Geometry: final body of the model. Coordinates: model frame, mm. A direction names the side the tool comes from. Give positions to 0.01 mm unless a question says otherwise; leave off trailing zeros. Write each loop counter-clockwise with the first axis right and the second up, starting at its lowest first coordinate (ties: lowest second). Pieces come first, ordered by that corner, then holes.
```python
from build123d import *

# Parameters (mm, degrees)
SKETCH_1_W          = 50
SKETCH_1_H          = 55
EXTRUDE_1_DEPTH     = 8
EXTRUDE_2_DEPTH     = 8
FILLET_1_R          = 8
CUT_EXTRUDE_1_DEPTH = 8
SKETCH_4_R          = 4
CUT_EXTRUDE_2_DEPTH = 8


with BuildPart() as part:
    # 草图1 → 凸台-拉伸1 (new body)
    with BuildSketch(Plane(origin=(0, 0, 0), x_dir=(0, 0, -1), z_dir=(1, 0, 0))):
        with Locations((0, 7.5)):
            Rectangle(SKETCH_1_W, SKETCH_1_H)
    extrude(amount=EXTRUDE_1_DEPTH)

    # 草图2 → 凸台-拉伸2 (add)
    with BuildSketch(Plane.XZ.offset(20)):
        Polygon((0, 25), (8, 25), (246.45, 25), (246.45, -25), (8, -25), (0, -25), align=None)
    extrude(amount=-EXTRUDE_2_DEPTH)

    # 圆角1
    fillet_1_edges = [part.edges().sort_by_distance(p)[0] for p in [
        (8, -12, 0),
    ]]
    fillet(fillet_1_edges, radius=FILLET_1_R)

    # 草图3 → 切除-拉伸1 (cut)
    with BuildSketch(Plane.XZ.offset(20)):
        with BuildLine():
            Line((176.45, -17.75), (226.45, -17.75))
            ThreePointArc((226.45, -17.75), (229.2, -15), (226.45, -12.25))
            Line((226.45, -12.25), (176.450000009, -12.25))
            ThreePointArc((176.450000009, -12.25), (173.7, -14.999999996), (176.45, -17.75))
        make_face()
        with BuildLine():
            Line((176.449999995, 12.25), (226.45, 12.25))
            ThreePointArc((226.45, 12.25), (229.2, 15), (226.45, 17.75))
            Line((226.45, 17.75), (176.45, 17.75))
            ThreePointArc((176.45, 17.75), (173.7, 15.000000003), (176.449999995, 12.25))
        make_face()
    extrude(amount=-CUT_EXTRUDE_1_DEPTH, mode=Mode.SUBTRACT)

    # 草图4 → 切除-拉伸2 (cut)
    with BuildSketch(Plane.ZY):
        with Locations((-15, 25)):
            Circle(SKETCH_4_R)
        with Locations((-15, 0)):
            Circle(SKETCH_4_R)
        with Locations((15, 25)):
            Circle(SKETCH_4_R)
        with Locations((15, 0)):
            Circle(SKETCH_4_R)
    extrude(amount=-CUT_EXTRUDE_2_DEPTH, mode=Mode.SUBTRACT)


solid = part.part
```
Item 1: Section D-D, the plane x = 114.5. Return the cut outline in (y, z).
Found:
outline: (-20, -25) - (-12, -25) - (-12, 25) - (-20, 25) - close
Item 2: Reachability of faces 1 (the face through (8, 16, 0)), 2 (the face through (173.7, -16.1, 15.1)), 3 (the face through (104, -13, -25)) from +Z, -Z, +X, -X, +Y, -Y: full face, straight path, thin tool, end or side. Return the list, or none.
Found:
face 1: +Z, -Z, +X, +Y
face 2: +Y, -Y
face 3: -Z, +X, -X, +Y, -Y
Item 3: Section A-A, the plane y = 25. Return the cut outline in (x, z), plus the area to 3 significant figures.
Found:
outline: (0, -25) - (8, -25) - (8, -19) - (0, -19) - close; (0, -11) - (8, -11) - (8, 11) - (0, 11) - close; (0, 19) - (8, 19) - (8, 25) - (0, 25) - close
area: 272 mm2
Item 4: Pin query (flat end, axial travel): pin 1 Ø5 at (y, z) = (25, -15) entering from +X; pin 2 Ø1.5 at (x, z) = (139, 9) entering from +Y; pin 3 Ø10.5 at (y, z) = (0, 15) entering from +X; pin 4 Ø1.5 at (y, z) = (25, 4.5) entering from +X. Return the tip coordinate at first contact, or that it passes through.
Found:
pin 1: passes through
pin 2: stops at y = -12
pin 3: stops at x = 8.1
pin 4: stops at x = 8
Item 5: Pull-direction query (Y, two-part tool) for faces 4 (the face through (125, -20, 0)), 5 (the face through (4, 0, 11)), 6 (the face through (106, -15, 25)); classes: +Y half, -Y half, draft (parallel to the pull), parting line (faces both ways), or undercut.
Found:
face 4: -Y half
face 5: undercut
face 6: draft
Item 6: Section B-B, the plane x = 194. Return the cut outline in (y, z), plus the area to 3 significant figures.
Found:
outline: (-20, -25) - (-12, -25) - (-12, -17.75) - (-20, -17.75) - close; (-20, -12.25) - (-12, -12.25) - (-12, 12.25) - (-20, 12.25) - close; (-20, 17.75) - (-12, 17.75) - (-12, 25) - (-20, 25) - close
area: 312 mm2
Item 7: Section C-C, the plane z = 5.5. Return the cut outline in (x, y), plus the area to 3 significant figures.
Found:
outline: (0, -20) - (246.45, -20) - (246.45, -12) - (16, -12) arc R8 cw to (8, -4) - (8, 35) - (0, 35) - close
area: 2,360 mm2
Item 8: Line query: L1, parallel to Y at x = 5.25, z = -15; L2, parallel to Z at x = 5.25, y = 0; L3, parallel to Z at x = 204, y = -16. Output: solid intervals per line, ascending.
Found:
L1: y = -20 to -4, 4 to 21, 29 to 35
L2: z = -25 to -19, -11 to 11, 19 to 25
L3: z = -25 to -17.75, -12.25 to 12.25, 17.75 to 25
